Geometry check sheet. Reference: the model listing, model coordinates, mm. A direction names the side the tool comes from. Give positions to 0.01 mm unless a question says otherwise; leave off trailing zeros. Order: outer loops, then holes, each group sorted by start corner. A loop starts at its lowest first (then second) coordinate and runs counter-clockwise, first axis right, second up. Notation, with made-up numbers: M -15.5,-12 L 0.5,-12 A23 ccw 0.5,12 Z; hole C -16,77.5 d11. An arc over 180 degrees is marked long. Answer as CSV lines item,"result".
from build123d import *

# Parameters (mm, degrees)
F0_R      = 63.5
F1_DEPTH  = 698.5
F3_R      = 44.45
F4_DEPTH  = 39.624
F4_FACE_R = 44.45
F1_FACE_R = 63.5


with BuildPart() as f1:
    # F0 (on Right) → F1 (new body, symmetric)
    with BuildSketch(Plane.YZ):
        Circle(F0_R)
    extrude(amount=F1_DEPTH, both=True)



with BuildPart() as f4:
    # F3 (on offset) → F4 (new body)
    with BuildSketch(Plane.YZ.offset(897.001)):
        Circle(F3_R)
    extrude(amount=-F4_DEPTH)


with BuildPart() as f1_1:
    add(f1.part)

    add(f4.part)  # F5 merges F4
    # F4_face (on face) → F5 section 0
    with BuildSketch(Plane(origin=(857.377, 0, 0), x_dir=(0, 1, 0), z_dir=(-1, 0, 0))):
        Circle(F4_FACE_R)
    # F1_face (on face) → F5 section 1
    with BuildSketch(Plane.YZ.offset(698.5)):
        Circle(F1_FACE_R)
    loft()

    # F6: F1 across plane


with BuildPart() as f1_2:
    add(f1_1.part)
    add(f1_1.part.mirror(Plane.YZ))


solid = f1_2.part
(1) Section check B-B on x = 654. Enter the section's corners in (y, z).
The answers:
outline,"C 0,0 d127"
(2) Tool access check on faces 1 (the face through (-877.466, 42.397, 13.352)), 2 (the face through (877.466, 42.397, 13.352)), 3 (the face through (897.001, -1, 1)). Record the directions out of +Z, -Z, +X, -X, +Y, -Y that give a thin tool (end or side, any length) a straight path to the whole face; none if there is none.
The answers:
face 1,"-X"
face 2,"+X"
face 3,"+Z, -Z, +X, +Y, -Y"
(3) Material ranges on line 1 (Z direction, x = -773, y = 31.5); line 2 (Z direction, x = -735.5, y = 17.5); line 3 (Y direction, x = -220, z = -8.5), recorded low to high.
The answers:
line 1,"z = -44.56 to 44.56"
line 2,"z = -56.41 to 56.41"
line 3,"y = -62.93 to 62.93"
(4) Gauge pin test, flat ends, axial feed: P1, Ø1.5, axis at x = -562, y = -33.5, coming from the +Z side; P2, Ø10, axis at x = -217.5, y = 5, coming from the -Z side; P3, Ø3, axis at x = 247, z = -34.5, coming from the -Y side. Record the tip position at first contact, or that the pin passes through.
The answers:
P1,"stops at z = 54.4"
P2,"stops at z = -63.5"
P3,"stops at y = -54.25"
(5) Section check A-A on y = 0. Enter the section's corners in (x, z), then the cut area to 3 significant figures.
The answers:
outline,"M -897,-44.45 L -857.38,-44.45 L -698.5,-63.5 L 698.5,-63.5 L 857.38,-44.45 L 897,-44.45 L 897,44.45 L 857.38,44.45 L 698.5,63.5 L -698.5,63.5 L -857.38,44.45 L -897,44.45 Z"
area,"219,000 mm2"
